from build123d import *

# Parameters (mm, degrees)
F0_W     = 35
F0_H     = 10
F2_DEPTH = 5
F0_W_2   = 5
F0_H_2   = 1.25
F3_DEPTH = 2.5
F4_R     = 0.25
F5_R     = 1
F6_R     = 0.5


with BuildPart() as f2:
    # F0 (on Top) → F2 (new body)
    with BuildSketch(Plane.XY):
        Rectangle(F0_W, F0_H)
        Polygon((-12.776, -2.25), (-12.776, 2.25), (-2.5, 2.25), (2.5, 2.25), (12.776, 2.25), (12.776, -2.25), (2.5, -2.25), (-2.5, -2.25), align=None, mode=Mode.SUBTRACT)
    extrude(amount=F2_DEPTH)

    # F0 (on Top) → F3 (join)
    with BuildSketch(Plane.XY):
        with Locations((0, 1.625)):
            Rectangle(F0_W_2, F0_H_2)
        with Locations((0, -1.625)):
            Rectangle(F0_W_2, F0_H_2)
    extrude(amount=F3_DEPTH)

    # F4
    f4_edges = [f2.edges().sort_by_distance(p)[0] for p in [
        (2.5, 1.625, 2.5),
        (0, 1, 2.5),
        (-2.5, 1.625, 2.5),
        (2.5, -1.625, 2.5),
        (-2.5, -1.625, 2.5),
        (0, -1, 2.5),
    ]]
    fillet(f4_edges, radius=F4_R)

    # F5
    f5_edges = [f2.edges().sort_by_distance(p)[0] for p in [
        (0, -5, 5),
        (0, 5, 5),
        (17.5, 0, 5),
        (-17.5, 0, 5),
    ]]
    fillet(f5_edges, radius=F5_R)

    # F6
    f6_edges = [f2.edges().sort_by_distance(p)[0] for p in [
        (0, 2.25, 5),
        (12.776, 0, 5),
        (0, -2.25, 5),
        (-12.776, 0, 5),
    ]]
    fillet(f6_edges, radius=F6_R)


solid = f2.part
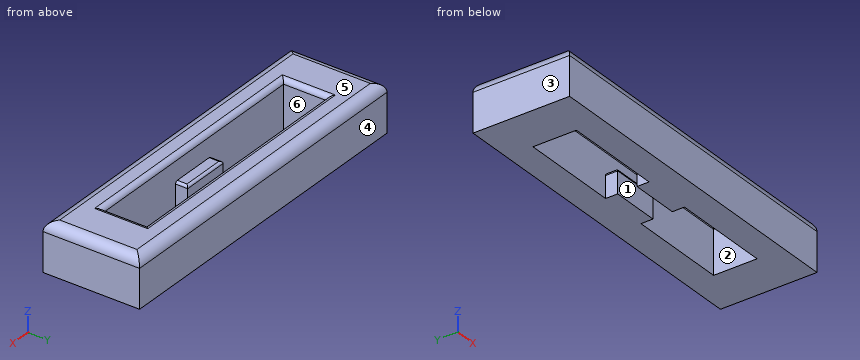
Can you work these out from the model? Positions are in its coordinate system, mm. Face numbers are marked on the shaded views. A direction names the side the tool comes from. Round coordinates to 2 decimals unless told otherwise and drop trailing zeros. Order: outer loops, then holes, each group sorted by start corner. A loop starts at its lowest first (then second) coordinate and runs counter-clockwise, first axis right, second up. Notation, with made-up numbers: M 65,87.5 L 100,87.5 A26 cw 100,119.5 Z; hole C 14,-23 d3. An arc over 180 degrees is marked long. Use a Markdown table: item, result.
1) Imagine slicing it at C-C (y = 0). List the corners of the cut face in (x, z) for me.
Geometry says:
| item | result |
|---|---|
| outline | M -17.5,0 L -12.78,0 L -12.78,4.5 A0.5 ccw -13.28,5 L -16.5,5 A1 ccw -17.5,4 Z; M 12.78,0 L 17.5,0 L 17.5,4 A1 ccw 16.5,5 L 13.28,5 A0.5 ccw 12.78,4.5 Z |
2) On a 3-axis mill with a long thin cutter (end or side, diameter ignored), from which of +Z, -Z, +X, -X, +Y, -Y can I reach the whole of each face in a straight line? I mean the marked faces 5 and 6. Say none if no direction works.
Geometry says:
| item | result |
|---|---|
| face 5 | +Z, +X, -X, +Y, -Y |
| face 6 | +Z, -Z |
3) Imagine slicing it at A-A (x = 1). List the corners of the cut face in (y, z) for me, then the cut area to 3 significant figures.
Geometry says:
| item | result |
|---|---|
| outline | M -5,0 L -1,0 L -1,2.25 A0.25 ccw -1.25,2.5 L -2.25,2.5 L -2.25,4.5 A0.5 ccw -2.75,5 L -4,5 A1 ccw -5,4 Z; M 1,0 L 5,0 L 5,4 A1 ccw 4,5 L 2.75,5 A0.5 ccw 2.25,4.5 L 2.25,2.5 L 1.25,2.5 A0.25 ccw 1,2.25 Z |
| area | 33.2 mm² |
4) Imagine slicing it at B-B (z = 1.3). List the corners of the cut face in (x, y) for me, then the cut area to 3 significant figures.
Geometry says:
| item | result |
|---|---|
| outline | M -17.5,-5 L 17.5,-5 L 17.5,5 L -17.5,5 Z; hole M -12.78,-2.25 L -2.5,-2.25 L -2.5,-1 L 2.5,-1 L 2.5,-2.25 L 12.78,-2.25 L 12.78,2.25 L 2.5,2.25 L 2.5,1 L -2.5,1 L -2.5,2.25 L -12.78,2.25 Z |
| area | 248 mm² |
5) If I drill on line 1 along X through (y, z) = (-1.75, 2.1); line 2 along X through (y, z) = (0.25, 0.95); line 3 along Y through (x, z) = (-10.5, 1.6), over which ranges is the centre line in solid material (lowest first)?
Geometry says:
| item | result |
|---|---|
| line 1 | x = -17.5 to -12.78, -2.5 to 2.5, 12.78 to 17.5 |
| line 2 | x = -17.5 to -12.78, 12.78 to 17.5 |
| line 3 | y = -5 to -2.25, 2.25 to 5 |
6) If we mould it in two halves opening along Y, with no side actions, what happens to the marked faces 1, 2, 3 and 4? For each: +Y half, -Y half, draft (parallel to the pull), parting line (faces both ways), or undercut.
Geometry says:
| item | result |
|---|---|
| face 1 | undercut |
| face 2 | undercut |
| face 3 | draft |
| face 4 | +Y half |
7) I'm going to push a flat-ended pin straight in: P1, Ø1.1, axis at x = 1, y = -1.5, coming from the +Z side. Where does the tip first touch, or does it pass through?
Geometry says:
| item | result |
|---|---|
| P1 | stops at z = 2.5 |
8) Imagine slicing it at D-D (z = 3.3). List the corners of the cut face in (x, y) for me.
Geometry says:
| item | result |
|---|---|
| outline | M -17.5,-5 L 17.5,-5 L 17.5,5 L -17.5,5 Z; hole M -12.78,-2.25 L 12.78,-2.25 L 12.78,2.25 L -12.78,2.25 Z |
